```python
from build123d import *

# Parameters (mm, degrees)
SKETCH1_W           = 45
SKETCH1_H           = 45
SKETCH1_R           = 11
SKETCH1_R_2         = 1.5
BOSS_EXTRUDE1_DEPTH = 3


with BuildPart() as part:
    # Sketch1 → Boss-Extrude1 (new body)
    with BuildSketch(Plane.XY):
        Rectangle(SKETCH1_W, SKETCH1_H)
        Polygon((20.15, -20.15), (20.15, -16.735786438), (20.15, 16.735786438), (16.735786438, 20.15), (-16.735786438, 20.15), (-20.15, 16.735786438), (-20.15, 16.077064234), (-20.15, -16.735786438), (-20.15, -20.15), (-16.735786438, -20.15), (16.735786438, -20.15), align=None, mode=Mode.SUBTRACT)
        Polygon((16.735786438, -20.15), (20.15, -20.15), (20.15, -16.735786438), (20.15, 16.735786438), (16.735786438, 20.15), (-16.735786438, 20.15), (-20.15, 16.735786438), (-20.15, 16.077064234), (-20.15, -16.735786438), (-20.15, -20.15), (-16.735786438, -20.15), align=None)
        Circle(SKETCH1_R, mode=Mode.SUBTRACT)
        with Locations((15.5, -15.5)):
            Circle(SKETCH1_R_2, mode=Mode.SUBTRACT)
        with Locations((15.5, 15.5)):
            Circle(SKETCH1_R_2, mode=Mode.SUBTRACT)
        with Locations((-15.5, -15.5)):
            Circle(SKETCH1_R_2, mode=Mode.SUBTRACT)
        with Locations((-15.5, 15.5)):
            Circle(SKETCH1_R_2, mode=Mode.SUBTRACT)
    extrude(amount=BOSS_EXTRUDE1_DEPTH)


solid = part.part
```
Build history of the part. All positions in model axes, mm. Round coordinates to 2 decimals unless told otherwise and drop trailing zeros. Loops run counter-clockwise (first coordinate to the right, second up) from the corner with the lowest first, then second, coordinate; pieces in that order, holes last.
Item 1: Pin check, flat tips, straight feed: P1, Ø2.5, axis at x = 15.5, y = -15.5, coming from the -Z side; P2, Ø12, axis at x = -2.5, y = 16.5, coming from the -Z side. Stop position of each tip, or through.
Item 2: Drill centre lines: line 1 along Y through (x, z) = (-15.5, 1.35); line 2 along X through (y, z) = (-14.5, 0.9); line 3 along X through (y, z) = (-9.5, 1.9). Where is each one in solid material? Low to high.
Item 3: Saw through at A-A (x = -15.5). List the corners of the cut face in (y, z), then the cut area to 3 significant figures.
Item 4: Saw through at D-D (y = 7). List the corners of the cut face in (x, z), then the cut area to 3 significant figures.
Item 5: Two-plate mould, pull along X, no slides. Class faces 1 (the face through (-17, 15.57, 1.48)), 2 (the face through (22.5, 0, 1)), 3 (the face through (-17, -15.43, 1.48)), 4 (the face through (0, 22.5, 1)): released by +X, released by -X, zero draft, split by the parting line, or undercut.
Item 6: Saw through at C-C (z = 2.5). List the corners of the cut face in (x, y), then the cut area to 3 significant figures.
Worked answers:
1. P1: passes through
1. P2: stops at z = 0
2. line 1: y = -22.5 to -17, -14 to 14, 17 to 22.5
2. line 2: x = -22.5 to -16.62, -14.38 to 14.38, 16.62 to 22.5
2. line 3: x = -22.5 to -5.55, 5.55 to 22.5
3. outline: (-22.5, 0) - (-17, 0) - (-17, 3) - (-22.5, 3) - close; (-14, 0) - (14, 0) - (14, 3) - (-14, 3) - close; (17, 0) - (22.5, 0) - (22.5, 3) - (17, 3) - close
3. area: 117 mm2
4. outline: (-22.5, 0) - (-8.49, 0) - (-8.49, 3) - (-22.5, 3) - close; (8.49, 0) - (22.5, 0) - (22.5, 3) - (8.49, 3) - close
4. area: 84.1 mm2
5. face 1: undercut
5. face 2: released by +X
5. face 3: undercut
5. face 4: zero draft
6. outline: (-22.5, -22.5) - (22.5, -22.5) - (22.5, 22.5) - (-22.5, 22.5) - close; hole circle Ø3 at (-15.5, -15.5); hole circle Ø3 at (-15.5, 15.5); hole circle Ø22 at (0, 0); hole circle Ø3 at (15.5, -15.5); hole circle Ø3 at (15.5, 15.5)
6. area: 1,620 mm2
